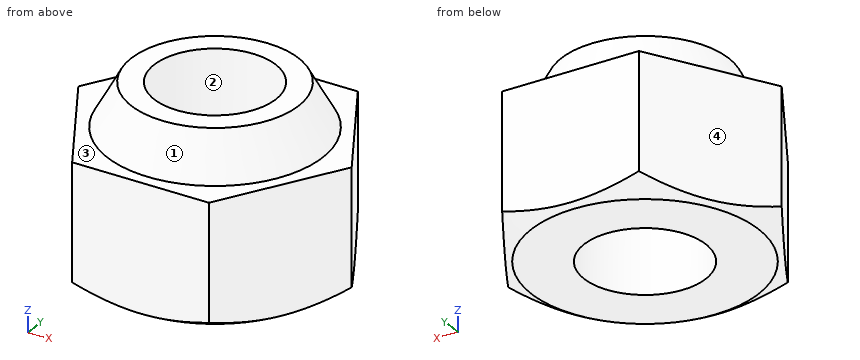
```python
from build123d import *

# Parameters (mm, degrees)
F_0186_EXTRUDE_DEPTH        = 3
F_0186_EXTRUDE_ROTATE_ANGLE = 120
F_0185_REVOLVE_ROTATE_ANGLE = 90
F_0188_CONE_ROTATE_ANGLE    = 90
F_0191_CYLINDER_SKETCH_R    = 1.4
F_0191_CYLINDER_DEPTH       = 10


with BuildPart() as part:
    # 0186_extrude_Sketch → 0186_extrude (new body)
    with BuildSketch(Plane.XY):
        Polygon((0, 0), (3.175426481, 0), (4.763139721, 2.75), (3.175426481, 5.5), (0, 5.5), (-1.58771324, 2.75), align=None)
    extrude(amount=F_0186_EXTRUDE_DEPTH)


with BuildPart() as part_1:
    # 0186_extrude_Rotate: moved
    add(part.part.rotate(Axis((0, 0, 0), (0, 0, 1)), F_0186_EXTRUDE_ROTATE_ANGLE))


with BuildPart() as part_2:
    # 0186_extrude_Translate: moved
    add(part_1.part.moved(Location((3.175426481, 0, 0))))


with BuildPart() as body_2:
    # 0185_revolve_Sketch → 0185_revolve (revolve)
    with BuildSketch(Plane.XY, mode=Mode.PRIVATE) as f_0185_revolve_sk:
        Polygon((0, 0), (2.6125, 0), (3.675426481, 0.61368089), (3.675426481, 3), (0, 3), align=None)
    revolve(f_0185_revolve_sk.sketch.rotate(Axis((0, -100, 0), (0, 1, 0)), 90), axis=Axis((0, -100, 0), (0, 1, 0)))


with BuildPart() as body_2_1:
    # 0185_revolve_Rotate: moved
    add(body_2.part.rotate(Axis((0, 0, 0), (1, 0, 0)), F_0185_REVOLVE_ROTATE_ANGLE))


with BuildPart() as part_3:
    add(part_2.part)

    # 0187_common: intersect body 2
    add(body_2_1.part, mode=Mode.INTERSECT)


with BuildPart() as body_2_2:
    # 0188_cone_Sketch → 0188_cone (revolve)
    with BuildSketch(Plane.XY, mode=Mode.PRIVATE) as f_0188_cone_sk:
        Polygon((0, 0), (2.475, 0), (1.925, 1), (0, 1), align=None)
    revolve(f_0188_cone_sk.sketch.rotate(Axis((0, -100, 0), (0, 1, 0)), 90), axis=Axis((0, -100, 0), (0, 1, 0)))


with BuildPart() as body_2_2_1:
    # 0188_cone_Rotate: moved
    add(body_2_2.part.rotate(Axis((0, 0, 0), (1, 0, 0)), F_0188_CONE_ROTATE_ANGLE))


with BuildPart() as body_2_2_2:
    # 0188_cone_Translate: moved
    add(body_2_2_1.part.moved(Location((0, 0, 3))))


with BuildPart() as part_4:
    add(part_3.part)

    # 0190_add: union body 2 2
    add(body_2_2_2.part)


with BuildPart() as body_2_3:
    # 0191_cylinder_Sketch → 0191_cylinder (new body)
    with BuildSketch(Plane.XY):
        Circle(F_0191_CYLINDER_SKETCH_R)
    extrude(amount=F_0191_CYLINDER_DEPTH)


with BuildPart() as body_2_3_1:
    # 0191_cylinder_Translate: moved
    add(body_2_3.part.moved(Location((0, 0, -5))))


with BuildPart() as part_5:
    add(part_4.part)

    # 0192_sub: cut body 2 3
    add(body_2_3_1.part, mode=Mode.SUBTRACT)


solid = part_5.part
```
Geometry: final body of the model. Coordinates: model frame, mm. Face numbers are marked on the shaded views. Round coordinates to 2 decimals unless told otherwise and drop trailing zeros. Order: outer loops, then holes, each group sorted by start corner. A loop starts at its lowest first (then second) coordinate and runs counter-clockwise, first axis right, second up. Notation, with made-up numbers: M 62.5,69 L 67.5,69 A5 ccw 67.5,73 Z; hole C -7,88.5 d8. An arc over 180 degrees is marked long. Use one line per item in the form item = value. Start each with the question number.
Q1. Cut plane B-B (z = 2.4). Return loops of the section in (x, y), and give its area (3 significant figures).
Q2. Mould query, pull axis X, two halves, no side actions, for the marked faces 1, 2, 3 and 4. Classes: +X half, -X half, draft (parallel to the pull), parting line (faces both ways), or undercut.
Q3. Material intervals for line 1 (Y direction, x = 0, z = 1.75); line 2 (Z direction, x = -2.5, y = -0.6); line 3 (X direction, y = 0.2, z = 3.15), sorted ascending. Write a range as [from, to].
Q4. Pin query (flat end, axial travel): pin 1 Ø1.7 at (x, y) = (0, 0) entering from +Z. Return the tip coordinate at first contact, or that it passes through.
Q5. Cut plane C-C (z = 3.65). Return loops of the section in (x, y) (1 decimal).
Geometry results:
q1.outline = M -3.18,0 L -1.59,-2.75 L 1.59,-2.75 L 3.18,0 L 1.59,2.75 L -1.59,2.75 Z; hole C 0,0 d2.8
q1.area = 20.0 mm^2
q2.face_1 = parting line
q2.face_2 = undercut
q2.face_3 = draft
q2.face_4 = -X half
q3.line_1 = [-2.75, -1.4], [1.4, 2.75]
q3.line_2 = [0, 3]
q3.line_3 = [-2.38, -1.39], [1.39, 2.38]
q4.pin_1 = through
q5.outline = C 0,0 d4.2; hole C 0,0 d2.8
